Part model, mm, in its own coordinate system. Face numbers are marked on the shaded views. A direction names the side the tool comes from. Round coordinates to 2 decimals unless told otherwise and drop trailing zeros. Write each loop counter-clockwise with the first axis right and the second up, starting at its lowest first coordinate (ties: lowest second). Pieces come first, ordered by that corner, then holes. Notation, with made-up numbers: M -7.75,36.5 L 51.25,36.5 A22 cw 51.25,42.5 Z; hole C -13,-13 d3. An arc over 180 degrees is marked long. Answer as a JSON object with one key per item and string values. Group by question number.
1. Two-plate mould, pull along Y, no slides. Class the marked faces 3 and 4: +Y half, -Y half, draft (parallel to the pull), parting line (faces both ways), or undercut.
2. Drill centre lines: line 1 (X direction, y = 23, z = 6); line 2 (X direction, y = -6, z = 5.5); line 3 (Y direction, x = 7.5, z = 3.25). Where is each one in solid material? Low to high. Write a range as from..to.
3. Band-saw the part on B-B, the plane y = 12. Write the cut outline in (x, z).
4. Drop flat-ended pins along their axis: pin 1 (1.5 mm diameter, centred on x = 30.5, z = 6, fed in from +Y); pin 2 (1 mm diameter, centred on x = -8, z = 3, fed in from -Y); pin 3 (3 mm diameter, centred on y = -7, z = 3, fed in from +X). Give the stop position or say it passes through.
5. Band-saw the part on C-C, the plane z = 3.5. Count the separate pieces of the cut face and the enclosed holes in it, plus the area to 3 significant figures.
6. Which spindle directions (+Z, -Z, +X, -X, +Y, -Y) get a long thin tool onto all of the face, cutting with end or side? Do the marked faces 1 and 2. Say none if no direction does.
7. Band-saw the part on A-A, the plane x = 11.5. Write the cut outline in (y, z).
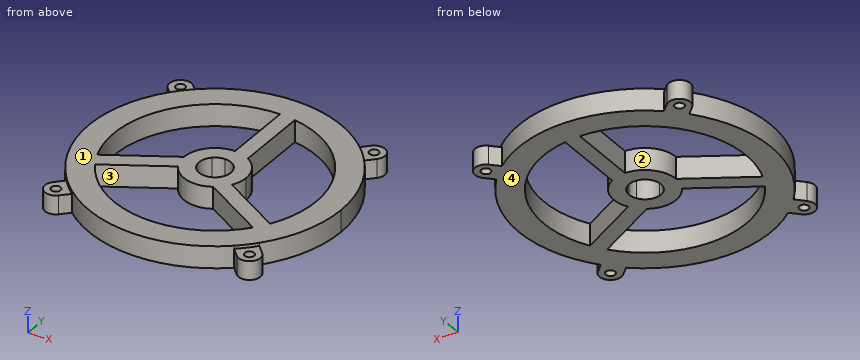
from build123d import *

# Parameters (mm, degrees)
F0_R     = 37
F1_DEPTH = 7
F0_R_2   = 1.5
F2_DEPTH = 6
F0_R_3   = 32.5
F3_DEPTH = 7
F5_DEPTH = 7


with BuildPart() as f1:
    # F0 (on Top) → F1 (new body)
    with BuildSketch(Plane.XY):
        with BuildLine():
            ThreePointArc((31.0055589695, -26.0558115012), (38.0524318426, -13.8658728851), (40.5, 0))
            ThreePointArc((40.5, 0), (38.0524318426, 13.8658728851), (31.0055589695, 26.0558115012))
            ThreePointArc((31.0055589695, 26.0558115012), (28.6378246381, 28.6378246381), (26.0558115012, 31.0055589695))
            ThreePointArc((26.0558115012, 31.0055589695), (0, 40.5), (-26.0558115012, 31.0055589695))
            ThreePointArc((-26.0558115012, 31.0055589695), (-28.6378246381, 28.6378246381), (-31.0055589695, 26.0558115012))
            ThreePointArc((-31.0055589695, 26.0558115012), (-40.5, 0), (-31.0055589695, -26.0558115012))
            ThreePointArc((-31.0055589695, -26.0558115012), (-28.6378246381, -28.6378246381), (-26.0558115012, -31.0055589695))
            ThreePointArc((-26.0558115012, -31.0055589695), (0, -40.5), (26.0558115012, -31.0055589695))
            ThreePointArc((26.0558115012, -31.0055589695), (28.6378246381, -28.6378246381), (31.0055589695, -26.0558115012))
        make_face()
        Circle(F0_R, mode=Mode.SUBTRACT)
    extrude(amount=F1_DEPTH)

    # F0 (on Top) → F2 (join)
    with BuildSketch(Plane.XY):
        with BuildLine():
            Line((-28.6378246381, -33.5875721064), (-26.0558115012, -31.0055589695))
            ThreePointArc((-26.0558115012, -31.0055589695), (-28.6378246381, -28.6378246381), (-31.0055589695, -26.0558115012))
            Line((-31.0055589695, -26.0558115012), (-33.5875721064, -28.6378246381))
            ThreePointArc((-33.5875721064, -28.6378246381), (-33.5875721064, -33.5875721064), (-28.6378246381, -33.5875721064))
        make_face()
        with Locations((-31.1126983722, -31.1126983722)):
            Circle(F0_R_2, mode=Mode.SUBTRACT)
        with BuildLine():
            Line((33.5875721064, -28.6378246381), (31.0055589695, -26.0558115012))
            ThreePointArc((31.0055589695, -26.0558115012), (28.6378246381, -28.6378246381), (26.0558115012, -31.0055589695))
            Line((26.0558115012, -31.0055589695), (28.6378246381, -33.5875721064))
            ThreePointArc((28.6378246381, -33.5875721064), (33.5875721064, -33.5875721064), (33.5875721064, -28.6378246381))
        make_face()
        with Locations((31.1126983722, -31.1126983722)):
            Circle(F0_R_2, mode=Mode.SUBTRACT)
        with BuildLine():
            ThreePointArc((26.0558115012, 31.0055589695), (28.6378246381, 28.6378246381), (31.0055589695, 26.0558115012))
            Line((31.0055589695, 26.0558115012), (33.5875721064, 28.6378246381))
            ThreePointArc((33.5875721064, 28.6378246381), (33.5875721064, 33.5875721064), (28.6378246381, 33.5875721064))
            Line((28.6378246381, 33.5875721064), (26.0558115012, 31.0055589695))
        make_face()
        with Locations((31.1126983722, 31.1126983722)):
            Circle(F0_R_2, mode=Mode.SUBTRACT)
        with BuildLine():
            ThreePointArc((-31.0055589695, 26.0558115012), (-28.6378246381, 28.6378246381), (-26.0558115012, 31.0055589695))
            Line((-26.0558115012, 31.0055589695), (-28.6378246381, 33.5875721064))
            ThreePointArc((-28.6378246381, 33.5875721064), (-33.5875721064, 33.5875721064), (-33.5875721064, 28.6378246381))
            Line((-33.5875721064, 28.6378246381), (-31.0055589695, 26.0558115012))
        make_face()
        with Locations((-31.1126983722, 31.1126983722)):
            Circle(F0_R_2, mode=Mode.SUBTRACT)
    extrude(amount=F2_DEPTH)

    # F0 (on Top) → F3 (join)
    with BuildSketch(Plane.XY):
        Circle(F0_R)
        Circle(F0_R_3, mode=Mode.SUBTRACT)
    extrude(amount=F3_DEPTH)

    # F4 (on face) → F5 (join)
    with BuildSketch(Plane.XY.offset(7)):
        with BuildLine():
            ThreePointArc((0, 10), (2.588190451, 9.6592582629), (5, 8.6602540378))
            Line((5, 8.6602540378), (5, 32.1130814467))
            ThreePointArc((5, 32.1130814467), (2.5074741258, 32.4031259836), (0, 32.5))
            Line((0, 32.5), (0, 10))
        make_face()
        with BuildLine():
            ThreePointArc((5, 1.0049875621), (5.0749384233, 0.5049752469), (5.1, 0))
            ThreePointArc((5.1, 0), (4.9262217141, -1.31997713), (4.4167295593, -2.55))
            Line((4.4167295593, -2.55), (8.6602540378, -5))
            ThreePointArc((8.6602540378, -5), (9.6592582629, -2.588190451), (10, 0))
            ThreePointArc((10, 0), (8.6602540378, 5), (5, 8.6602540378))
            Line((5, 8.6602540378), (5, 1.0049875621))
        make_face()
        with BuildLine():
            ThreePointArc((0, 5.1), (3.2314519518, 3.9455947946), (5, 1.0049875621))
            Line((5, 1.0049875621), (5, 8.6602540378))
            ThreePointArc((5, 8.6602540378), (2.588190451, 9.6592582629), (0, 10))
            Line((0, 10), (0, 5.1))
        make_face()
        with BuildLine():
            ThreePointArc((-3.3703447593, 3.8276332379), (-1.8012593493, 4.7713168787), (0, 5.1))
            Line((0, 5.1), (0, 10))
            ThreePointArc((0, 10), (-7.0710678119, 7.0710678119), (-10, 0))
            Line((-10, 0), (-3.3703447593, 3.8276332379))
        make_face()
        with BuildLine():
            ThreePointArc((-4.4167295593, -2.55), (-5.0327113011, 0.825722084), (-3.3703447593, 3.8276332379))
            Line((-3.3703447593, 3.8276332379), (-10, 0))
            ThreePointArc((-10, 0), (-9.6592582629, -2.588190451), (-8.6602540378, -5))
            Line((-8.6602540378, -5), (-4.4167295593, -2.55))
        make_face()
        with BuildLine():
            Line((5, -8.6602540378), (-1.6296552407, -4.8326208))
            ThreePointArc((-1.6296552407, -4.8326208), (-3.2314519518, -3.9455947946), (-4.4167295593, -2.55))
            Line((-4.4167295593, -2.55), (-8.6602540378, -5))
            ThreePointArc((-8.6602540378, -5), (-2.588190451, -9.6592582629), (5, -8.6602540378))
        make_face()
        with BuildLine():
            Line((8.6602540378, -5), (4.4167295593, -2.55))
            ThreePointArc((4.4167295593, -2.55), (1.8012593493, -4.7713168787), (-1.6296552407, -4.8326208))
            Line((-1.6296552407, -4.8326208), (5, -8.6602540378))
            ThreePointArc((5, -8.6602540378), (7.0710678119, -7.0710678119), (8.6602540378, -5))
        make_face()
        with BuildLine():
            Line((28.145825623, -16.25), (8.6602540378, -5))
            ThreePointArc((8.6602540378, -5), (7.0710678119, -7.0710678119), (5, -8.6602540378))
            Line((5, -8.6602540378), (25.3107443266, -20.3866677423))
            ThreePointArc((25.3107443266, -20.3866677423), (26.8081932009, -18.3730992841), (28.145825623, -16.25))
        make_face()
        with BuildLine():
            ThreePointArc((-8.6602540378, -5), (-9.6592582629, -2.588190451), (-10, 0))
            Line((-10, 0), (-30.3107443266, -11.7264137044))
            ThreePointArc((-30.3107443266, -11.7264137044), (-29.3156673267, -14.0300266995), (-28.145825623, -16.25))
            Line((-28.145825623, -16.25), (-8.6602540378, -5))
        make_face()
    extrude(amount=-F5_DEPTH)


solid = f1.part
Worked answers:
{
 "1": {"face 3": "undercut", "face 4": "draft"},
 "2": {"line 1": "x = -33.34..-22.96, 0..5, 22.96..33.34", "line 2": "x = -40.05..-31.94, -20.39..-10.39, -8..10.39, 31.94..40.05", "line 3": "y = -39.8..-31.62, -10.1..6.61, 31.62..39.8"},
 "3": {"outline": "M -38.68,0 L -30.2,0 L -30.2,7 L -38.68,7 Z; M 0,0 L 5,0 L 5,7 L 0,7 Z; M 30.2,0 L 38.68,0 L 38.68,7 L 30.2,7 Z"},
 "4": {"pin 1": "stops at y = 34.61", "pin 2": "stops at y = -39.8", "pin 3": "stops at x = 40.12"},
 "5": {"separate pieces": "1", "enclosed holes": "8", "area": "2,560 mm^2"},
 "6": {"face 1": "+Z, +X, -X, +Y, -Y", "face 2": "+Z, -Z"},
 "7": {"outline": "M -38.83,0 L -30.4,0 L -30.4,7 L -38.83,7 Z; M -12.41,0 L -6.64,0 L -6.64,7 L -12.41,7 Z; M 30.4,0 L 38.83,0 L 38.83,7 L 30.4,7 Z"}
}
